Part model, mm, in its own coordinate system. Round coordinates to 2 decimals unless told otherwise and drop trailing zeros. Write each loop counter-clockwise with the first axis right and the second up, starting at its lowest first coordinate (ties: lowest second). Pieces come first, ordered by that corner, then holes. Notation, with made-up numbers: M -24,83 L 4,83 A23 ccw 4,116 Z; hole C 59,-2 d8. An arc over 180 degrees is marked long. Answer as a JSON object with one key per item and string values. Group by question number.
1. Band-saw the part on D-D, the plane y = -20. Write the cut outline in (x, z).
2. Band-saw the part on B-B, the plane z = -53.5. Write the cut outline in (x, y), plus the area to 3 significant figures.
3. Drill centre lines: line 1 (Z direction, x = 2.6, y = -21); line 2 (Y direction, x = 0.8, z = -102.5); line 3 (Y direction, x = 2.45, z = -95). Where is each one in solid material? Low to high. Write a range as from..to.
4. Drop flat-ended pins along their axis: pin 1 (1.5 mm diameter, centred on x = 1.5, z = -72, fed in from +Y); pin 2 (0.9 mm diameter, centred on x = 2, y = -39, fed in from +Z); pin 3 (0.8 mm diameter, centred on x = 1, y = -11.5, fed in from +Z). Give the stop position or say it passes through.
5. Band-saw the part on C-C, the plane y = 29.5. Write the cut outline in (x, z), plus the area to 3 significant figures.
6. Band-saw the part on A-A, the plane z = -95. Write the cut outline in (x, y), plus the area to 4 significant figures.
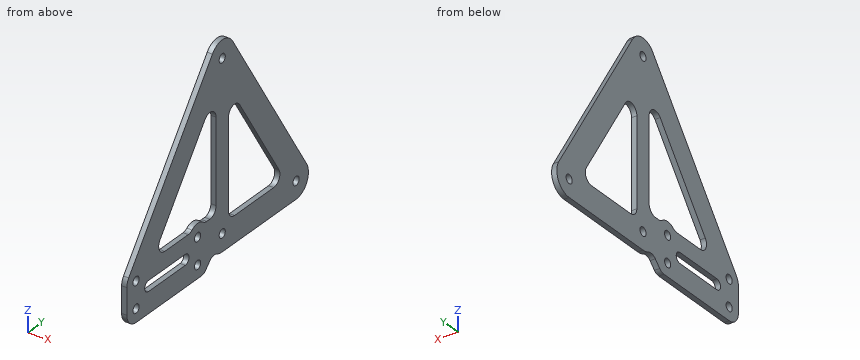
from build123d import *

# Parameters (mm, degrees)
SKETCH_1_R      = 2.5
EXTRUDE_1_DEPTH = 3


with BuildPart() as part:
    # 草图1 → 凸台-拉伸1 (new body)
    with BuildSketch(Plane(origin=(0, 0, 0), x_dir=(0, 0, -1), z_dir=(1, 0, 0))):
        with BuildLine():
            Line((-5.339929914, 8.45488903), (89.660070086, 68.45488903))
            ThreePointArc((89.660070086, 68.45488903), (99.827043653, 68.757833612), (105, 60))
            Line((105, 60), (105, 0))
            ThreePointArc((105, 0), (104.752868622, -2.209423827), (104.023689271, -4.309644063))
            ThreePointArc((104.023689271, -4.309644063), (103.607541108, -7.309975988), (105, -10))
            Line((105, -10), (108.535533906, -13.535533906))
            ThreePointArc((108.535533906, -13.535533906), (109.619397663, -15.15765065), (110, -17.071067812))
            Line((110, -17.071067812), (110, -70))
            ThreePointArc((110, -70), (107.803300859, -75.303300859), (102.5, -77.5))
            Line((102.5, -77.5), (87.5, -77.5))
            ThreePointArc((87.5, -77.5), (85.096555547, -77.10446724), (82.946615365, -75.959587936))
            Line((82.946615365, -75.959587936), (-6.071179513, -7.946117248))
            ThreePointArc((-6.071179513, -7.946117248), (-9.990075391, 0.44541405), (-5.339929914, 8.45488903))
        make_face()
        Circle(SKETCH_1_R, mode=Mode.SUBTRACT)
        with Locations((95, 0)):
            Circle(SKETCH_1_R, mode=Mode.SUBTRACT)
        with Locations((95, 60)):
            Circle(SKETCH_1_R, mode=Mode.SUBTRACT)
        with Locations((87.5, -20)):
            Circle(SKETCH_1_R, mode=Mode.SUBTRACT)
        with Locations((102.5, -20)):
            Circle(SKETCH_1_R, mode=Mode.SUBTRACT)
        with Locations((87.5, -70)):
            Circle(SKETCH_1_R, mode=Mode.SUBTRACT)
        with Locations((102.5, -70)):
            Circle(SKETCH_1_R, mode=Mode.SUBTRACT)
        with BuildLine():
            Line((82.330035043, 46.084178697), (31.890205922, 14.227444515))
            ThreePointArc((31.890205922, 14.227444515), (29.757191461, 8.610255883), (34.560170879, 5))
            Line((34.560170879, 5), (85, 5))
            ThreePointArc((85, 5), (88.535533906, 6.464466094), (90, 10))
            Line((90, 10), (90, 41.856734182))
            ThreePointArc((90, 41.856734182), (87.413521827, 46.235650988), (82.330035043, 46.084178697))
        make_face(mode=Mode.SUBTRACT)
        with BuildLine():
            Line((29.559523335, -5), (77.5, -5))
            ThreePointArc((77.5, -5), (81.035533906, -6.464466094), (82.5, -10))
            Line((82.5, -10), (82.5, -12.5))
            ThreePointArc((82.5, -12.5), (82.24341649, -14.08113883), (81.5, -15.5))
            ThreePointArc((81.5, -15.5), (80, -20), (81.5, -24.5))
            ThreePointArc((81.5, -24.5), (82.24341649, -25.91886117), (82.5, -27.5))
            Line((82.5, -27.5), (82.5, -46.628611267))
            ThreePointArc((82.5, -46.628611267), (79.716083394, -51.110683822), (74.464410244, -50.601669891))
            Line((74.464410244, -50.601669891), (26.523933579, -13.973058624))
            ThreePointArc((26.523933579, -13.973058624), (24.823211842, -8.397703698), (29.559523335, -5))
        make_face(mode=Mode.SUBTRACT)
        with BuildLine():
            Line((98, -30), (98, -60))
            ThreePointArc((98, -60), (95, -63), (92, -60))
            Line((92, -60), (92, -30))
            ThreePointArc((92, -30), (95, -27), (98, -30))
        make_face(mode=Mode.SUBTRACT)
    extrude(amount=EXTRUDE_1_DEPTH)


solid = part.part
Worked answers:
{
 "1": {"outline": "M 0,-110 L 3,-110 L 3,-105 L 0,-105 Z; M 0,-100 L 3,-100 L 3,-90 L 0,-90 Z; M 0,-85 L 3,-85 L 3,-80 L 0,-80 Z; M 0,-34.41 L 3,-34.41 L 3,-9.71 L 0,-9.71 Z"},
 "2": {"outline": "M 0,-53.46 L 3,-53.46 L 3,-34.58 L 0,-34.58 Z; M 0,-5 L 3,-5 L 3,5 L 0,5 Z; M 0,27.88 L 3,27.88 L 3,45.62 L 0,45.62 Z", "area": "140 mm^2"},
 "3": {"line 1": "z = -110..-104.79, -100.21..-89.79, -85.21..-80.07, -35.72..-11.01", "line 2": "y = -77.5..-72.5, -67.5..-22.5, -17.5..66.61", "line 3": "y = -77.5..-63, -27..-2.5, 2.5..57.5, 62.5..70"},
 "4": {"pin 1": "stops at y = 57.77", "pin 2": "stops at z = -33.98", "pin 3": "stops at z = 1.94"},
 "5": {"outline": "M 0,-105 L 3,-105 L 3,-90 L 0,-90 Z; M 0,-56.07 L 3,-56.07 L 3,-27.98 L 0,-27.98 Z", "area": "129 mm^2"},
 "6": {"outline": "M 0,-77.5 L 3,-77.5 L 3,-63 L 0,-63 Z; M 0,-27 L 3,-27 L 3,-2.5 L 0,-2.5 Z; M 0,2.5 L 3,2.5 L 3,57.5 L 0,57.5 Z; M 0,62.5 L 3,62.5 L 3,70 L 0,70 Z", "area": "304.5 mm^2"}
}
